```python
from build123d import *

# Parameters (mm, degrees)
RESSALTO_EXTRUS_O1_DEPTH = 40
ESBO_O4_R                = 7.8
CORTE_EXTRUS_O1_DEPTH    = 61
CORTE_EXTRUS_O2_DEPTH    = 3
FILETE2_R                = 3
CORTE_EXTRUS_O5_DEPTH    = 61
ESBO_O10_R               = 2.5
CORTE_EXTRUS_O6_DEPTH    = 38
ESBO_O11_R               = 4.25
CORTE_EXTRUS_O7_DEPTH    = 30
CORTE_EXTRUS_O8_DEPTH    = 30
ESBO_O13_W               = 2
ESBO_O13_H               = 5
RESSALTO_EXTRUS_O2_DEPTH = 5


with BuildPart() as part:
    # Esboço2 → Ressalto-extrusão1 (new body)
    with BuildSketch(Plane.XY):
        with BuildLine():
            Line((-246.218768802, 113.822486613), (-237.781231198, 113.822486613))
            Line((-237.781231198, 113.822486613), (-201.966801004, 113.822486613))
            Line((-201.966801004, 113.822486613), (-194.033198996, 113.822486613))
            Line((-194.033198996, 113.822486613), (-190, 113.822486613))
            Line((-190, 113.822486613), (-190, 138.123568891))
            Line((-190, 138.123568891), (-190, 163.212189341))
            ThreePointArc((-190, 163.212189341), (-191.464466094, 166.747723246), (-195, 168.212189341))
            Line((-195, 168.212189341), (-245, 168.212189341))
            ThreePointArc((-245, 168.212189341), (-248.535533906, 166.747723246), (-250, 163.212189341))
            Line((-250, 163.212189341), (-250, 138.123568891))
            Line((-250, 138.123568891), (-250, 113.822486613))
            Line((-250, 113.822486613), (-246.218768802, 113.822486613))
        make_face()
    extrude(amount=RESSALTO_EXTRUS_O1_DEPTH)

    # Esboço4 → Corte-extrusão1 (cut, through all)
    with BuildSketch(Plane(origin=(-190, 0, 0), x_dir=(0, 0, -1), z_dir=(1, 0, 0))):
        with Locations((-11.90241208, 122.212171493)):
            Circle(ESBO_O4_R)
        with Locations((-28.90241208, 122.212171493)):
            Circle(ESBO_O4_R)
    extrude(amount=-CORTE_EXTRUS_O1_DEPTH, mode=Mode.SUBTRACT)

    # Esboço5 → Corte-extrusão2 (cut)
    with BuildSketch(Plane(origin=(0, 0, 0), x_dir=(-1, 0, 0), z_dir=(0, 0, -1))):
        with BuildLine():
            Line((190, 163.212189341), (190, 113.822486613))
            Line((190, 113.822486613), (250, 113.822486613))
            Line((250, 113.822486613), (250, 163.212189341))
            ThreePointArc((250, 163.212189341), (248.535533906, 166.747723246), (245, 168.212189341))
            Line((245, 168.212189341), (195, 168.212189341))
            ThreePointArc((195, 168.212189341), (191.464466094, 166.747723246), (190, 163.212189341))
        make_face()
    extrude(amount=-CORTE_EXTRUS_O2_DEPTH, mode=Mode.SUBTRACT)

    # Filete2
    filete2_edges = [part.edges().sort_by_distance(p)[0] for p in [
        (-220, 113.822486613, 40),
        (-220, 113.822486613, 3),
    ]]
    fillet(filete2_edges, radius=FILETE2_R)

    # Esboço8 → Corte-extrusão5 (cut, through all)
    with BuildSketch(Plane.ZY.offset(250)):
        Polygon((23.874860756, 142.212171493), (23.874860756, 152.212171493), (23.874860756, 182.191519565), (13.874860756, 182.191519565), (13.874860756, 152.212171493), (13.874860756, 142.212171493), align=None)
    extrude(amount=-CORTE_EXTRUS_O5_DEPTH, mode=Mode.SUBTRACT)

    # Esboço10 → Corte-extrusão6 (cut, through all)
    with BuildSketch(Plane.XY.offset(40)):
        with Locations((-210, 160.173107934)):
            Circle(ESBO_O10_R)
        with Locations((-230, 160.173107934)):
            Circle(ESBO_O10_R)
    extrude(amount=-CORTE_EXTRUS_O6_DEPTH, mode=Mode.SUBTRACT)

    # Esboço11 → Corte-extrusão7 (cut)
    with BuildSketch(Plane(origin=(0, 168.212189341, 0), x_dir=(1, 0, 0), z_dir=(0, 1, 0))):
        with Locations((-199.5, -8.5)):
            Circle(ESBO_O11_R)
        with Locations((-240.5, -8.5)):
            Circle(ESBO_O11_R)
    extrude(amount=-CORTE_EXTRUS_O7_DEPTH, mode=Mode.SUBTRACT)

    # Esboço12 → Corte-extrusão8 (cut)
    with BuildSketch(Plane.ZY.offset(250)):
        Polygon((27.874860756, 152.212171493), (27.874860756, 142.212171493), (37.874860756, 142.212171493), (37.874860756, 152.212171493), (37.874860756, 170.639409053), (27.874860756, 170.639409053), align=None)
    extrude(amount=-CORTE_EXTRUS_O8_DEPTH, mode=Mode.SUBTRACT)


with BuildPart() as body_2:
    # Espelhar1: mirrored copy
    add(part.part.mirror(Plane(origin=(-245, 168.212189341, 40), x_dir=(0, 0, 1), z_dir=(0, -1, 0))))

    # Esboço13 → Ressalto-extrusão2 (add)
    with BuildSketch(Plane.ZY.offset(250)):
        with Locations((16.72, 203.212207189)):
            Rectangle(ESBO_O13_W, ESBO_O13_H)
    extrude(amount=RESSALTO_EXTRUS_O2_DEPTH)


solid = body_2.part
```
Geometry check sheet. Reference: the model listing, model coordinates, mm. A direction names the side the tool comes from. Round coordinates to 2 decimals unless told otherwise and drop trailing zeros. Loops run counter-clockwise (first coordinate to the right, second up) from the corner with the lowest first, then second, coordinate; pieces in that order, holes last. Notation, with made-up numbers: (5.25, -4.75) - (32.25, -4.75) arc R15 cw to (32.25, 9.25) - close; hole circle Ø11 at (64, 15.25). An arc over 180 degrees is marked (long way). Use a Markdown table: item, result.
Q1. Material ranges on line 1 (X direction, y = 196, z = 8.5); line 2 (Y direction, x = -210, z = 36); line 3 (Z direction, x = -235.5, y = 181), recorded low to high.
Solutions:
| item | result |
|---|---|
| line 1 | x = -250 to -244.75, -236.25 to -203.75, -195.25 to -190 |
| line 2 | y = 168.21 to 173.75, 178.75 to 210.98, 217.45 to 222.6 |
| line 3 | z = 3 to 13.87, 23.87 to 27.87, 37.87 to 40 |
Q2. Cross-section at A-A on y = 182. Record the cut outline in (x, z), plus the area to 3 significant figures.
Solutions:
| item | result |
|---|---|
| outline | (-250, 3) - (-190, 3) - (-190, 13.87) - (-250, 13.87) - close; (-250, 23.87) - (-190, 23.87) - (-190, 40) - (-250, 40) - (-250, 37.87) - (-220, 37.87) - (-220, 27.87) - (-250, 27.87) - close; hole circle Ø8.5 at (-240.5, 8.5); hole circle Ø8.5 at (-199.5, 8.5) |
| area | 1,210 mm2 |
Q3. Cross-section at B-B on z = 29. Record the cut outline in (x, y), plus the area to 3 significant figures.
Solutions:
| item | result |
|---|---|
| outline | (-250, 194.21) - (-220, 194.21) - (-220, 168.21) - (-195, 168.21) arc R5 ccw to (-190, 173.21) - (-190, 206.41) - (-250, 206.41) - close; (-250, 222.01) - (-190, 222.01) - (-190, 222.6) - (-250, 222.6) - close; hole circle Ø5 at (-210, 176.25) |
| area | 1,520 mm2 |
Q4. Cross-section at D-D on y = 209. Record the cut outline in (x, z).
Solutions:
| item | result |
|---|---|
| outline | (-250, 3) - (-190, 3) - (-190, 6.1) - (-250, 6.1) - close; (-250, 17.71) - (-190, 17.71) - (-190, 23.1) - (-250, 23.1) - close; (-250, 34.71) - (-190, 34.71) - (-190, 40) - (-250, 40) - close |
Q5. Access from +Z, -Z, +X, -X, +Y, -Y to the whole of each face (thin tool, end or side, straight path). Record for faces 4 (the flat face through (-235, 181, 37.875)), 5 (the cylindrical face through (-202.87, 183, 11.09)), 6 (the flat face through (-252, 203, 15.72)).
Solutions:
| item | result |
|---|---|
| face 4 | -X, -Y |
| face 5 | -Y |
| face 6 | -Z, -X, +Y, -Y |
Q6. Cross-section at C-C on x = -230. Record the cut outline in (y, z).
Solutions:
| item | result |
|---|---|
| outline | (168.21, 3) - (173.75, 3) - (173.75, 13.87) - (168.21, 13.87) - close; (168.21, 23.87) - (173.75, 23.87) - (173.75, 27.87) - (168.21, 27.87) - close; (168.21, 37.87) - (173.75, 37.87) - (173.75, 40) - (168.21, 40) - close; (178.75, 3) - (219.6, 3) arc R3 ccw to (222.6, 6) - (222.6, 37) arc R3 ccw to (219.6, 40) - (178.75, 40) - (178.75, 37.87) - (194.21, 37.87) - (194.21, 27.87) - (178.75, 27.87) - (178.75, 23.87) - (194.21, 23.87) - (194.21, 13.87) - (178.75, 13.87) - close; hole circle Ø15.6 at (214.21, 11.9); hole circle Ø15.6 at (214.21, 28.9) |
Q7. Go/stop test with flat-tipped pins: P1, Ø9.5, axis at x = -198.5, z = 9, coming from the -Y side; P2, Ø4.5, axis at x = -230, y = 176.25, coming from the -Z side; P3, Ø2, axis at x = -223.5, z = 29, coming from the -Y side; P4, Ø2, axis at x = -253.5, z = 16.5, coming from the -Y side. Record where each tip stops, or that it passes through.
Solutions:
| item | result |
|---|---|
| P1 | stops at y = 168.21 |
| P2 | passes through |
| P3 | stops at y = 194.21 |
| P4 | stops at y = 200.71 |
Q8. Draft check along Z on faces 1 (the cylindrical face through (-191.426, 169.716, 8.361)), 2 (the flat face through (-220, 181, 23.875)), 3 (the cylindrical face through (-219.58, 221.7, 39.145)). Enter one of: released by +Z, released by -Z, zero draft, split by the parting line, or undercut.
Solutions:
| item | result |
|---|---|
| face 1 | zero draft |
| face 2 | undercut |
| face 3 | released by +Z |
